Here's the drawing with two shaded views (mm, measured from the low corner). I have some questions. A direction names the side the tool comes from. Coordinates: 2 decimals unless noted, no trailing zeros. Write each loop counter-clockwise with the first axis right and the second up, starting at its lowest first coordinate (ties: lowest second). Pieces come first, ordered by that corner, then holes.
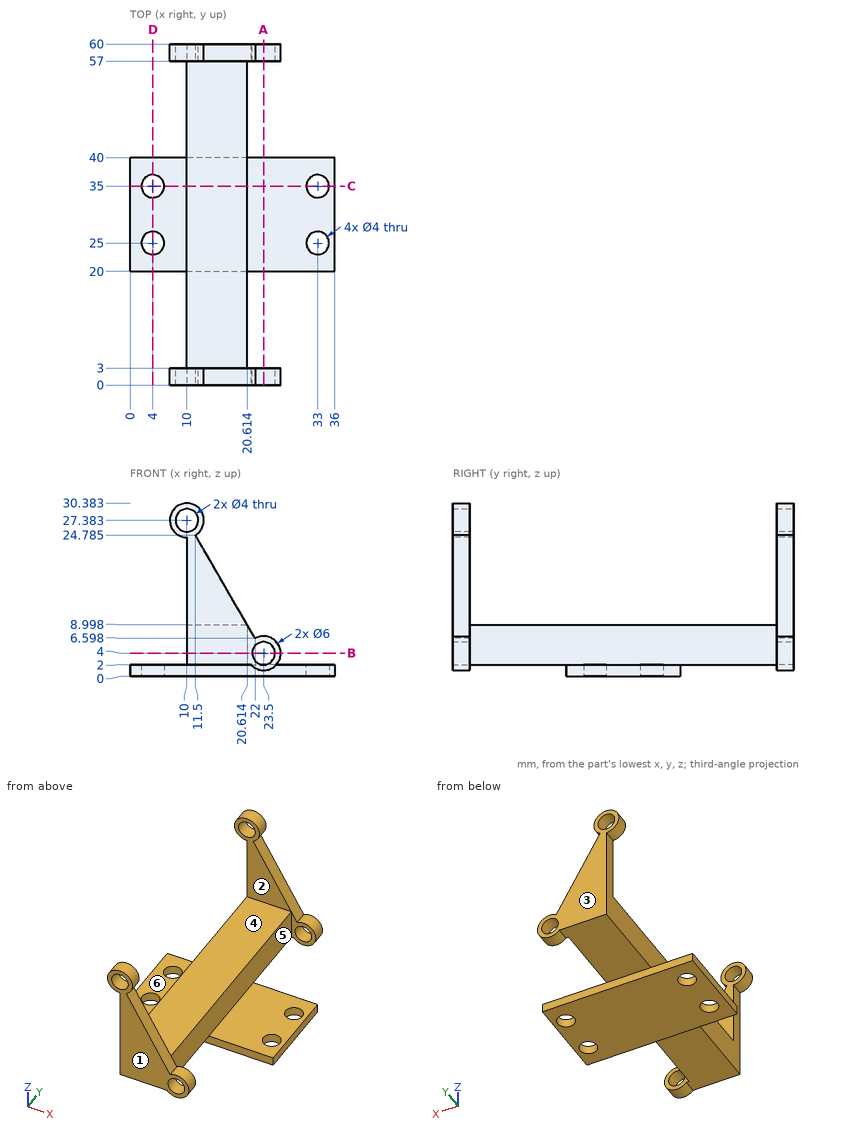
1. If we mould it in two halves opening along Y, with no side actions, what happens to the marked faces 1, 2 and 3? For each: pulls with the +Y half, pulls with the -Y half, needs draft (parallel to the pull), parting line crosses it, or undercut.
Verdict:
face 1: pulls with the -Y half
face 2: undercut
face 3: pulls with the +Y half
2. I want a section at A-A on x = 23.5. Please give me the cut outline in (y, z).
Verdict:
outline: (0, 1) - (3, 1) - (3, 2) - (0, 2) - close; (0, 6) - (3, 6) - (3, 7) - (0, 7) - close; (20, 0) - (40, 0) - (40, 2) - (20, 2) - close; (57, 1) - (60, 1) - (60, 2) - (57, 2) - close; (57, 6) - (60, 6) - (60, 7) - (57, 7) - close
3. On a 3-axis mill with a long thin cutter (end or side, diameter ignored), from which of +Z, -Z, +X, -X, +Y, -Y can I reach the whole of each face in a straight line? I mean the marked faces 4, 5 and 6. Say none if no direction works.
Verdict:
face 4: +Z, +X, -X
face 5: +Z, +X
face 6: +Z, -X, +Y, -Y
4. Please list where these lines run through material, in increasing order: line 1 along Y through (x, z) = (4, 1.4); line 2 along X through (y, z) = (58, 4); line 3 along X through (y, z) = (21, 2.5) (1 decimal).
Verdict:
line 1: y = 20 to 23, 27 to 33, 37 to 40
line 2: x = 10 to 21.5, 25.5 to 26.5
line 3: x = 10 to 20.6
5. I want a section at D-D on x = 4. Please give me the cut outline in (y, z), plus the area to 3 significant figures.
Verdict:
outline: (20, 0) - (23, 0) - (23, 2) - (20, 2) - close; (27, 0) - (33, 0) - (33, 2) - (27, 2) - close; (37, 0) - (40, 0) - (40, 2) - (37, 2) - close
area: 24.0 mm2
6. I want a section at C-C on y = 35. Please give me the cut outline in (x, z) (1 decimal).
Verdict:
outline: (0, 0) - (2, 0) - (2, 2) - (0, 2) - close; (6, 0) - (31, 0) - (31, 2) - (20.6, 2) - (20.6, 9) - (10, 9) - (10, 2) - (6, 2) - close; (35, 0) - (36, 0) - (36, 2) - (35, 2) - close
7. I want a section at B-B on z = 4. Please give me the cut outline in (x, y) (1 decimal).
Verdict:
outline: (10, 0) - (21.5, 0) - (21.5, 3) - (20.6, 3) - (20.6, 57) - (21.5, 57) - (21.5, 60) - (10, 60) - close; (25.5, 0) - (26.5, 0) - (26.5, 3) - (25.5, 3) - close; (25.5, 57) - (26.5, 57) - (26.5, 60) - (25.5, 60) - close
8. For pin 1 (5.5 mm diameter, centred on x = 16.5, y = 9, fed in from -Z); pin 2 (10 mm diameter, centred on y = 48.5, z = 6.5, fed in from +X); pin 3 (4.5 mm diameter, centred on x = 10, z = 27.38, fed in from -Y); pin 4 (3 mm diameter, centred on x = 10, z = 27.38, fed in from -Y), each with a flat end and sliding along its axis, tell me the tip position at first contact or that it passes through.
Verdict:
pin 1: stops at z = 2
pin 2: stops at x = 20.61
pin 3: stops at y = 0
pin 4: passes through
